Design review of the part shown in the three views and the two pictorial views. Dimensions are in mm from the part's minimum x, y and z. A direction names the side the tool comes from. Coordinates: 2 decimals unless noted, no trailing zeros. Write each loop counter-clockwise with the first axis right and the second up, starting at its lowest first coordinate (ties: lowest second). Pieces come first, ordered by that corner, then holes. Notation, with made-up numbers: M -36.75,10.5 L 0.25,10.5 A28 cw 0.25,33.5 Z; hole C 17,29.5 d5. An arc over 180 degrees is marked long. Answer as a JSON object with one key per item and string values.
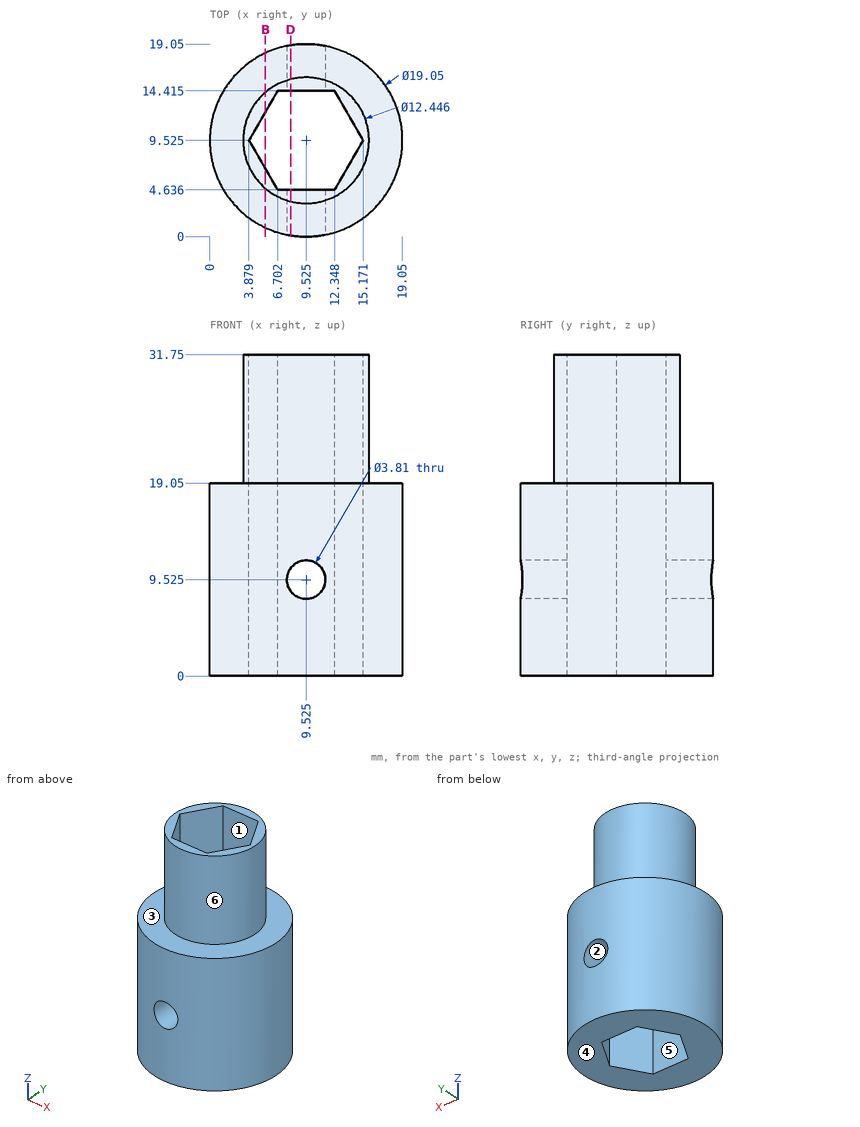
(1) Add section D-D on x = 8. Count the separate pieces of the cut face and the enclosed holes in it.
Results list:
{"separate pieces": "4", "enclosed holes": "0"}
(2) For pin 1 Ø6 at (y, z) = (2, 15) entering from -X; pin 2 Ø1 at (x, z) = (10.5, 5) entering from -Y; pin 3 Ø6 at (y, z) = (4, 18.5) entering from +X, all flat-tipped, find the tip position at first contact; note any pin that passes through.
Results list:
{"pin 1": "x = 1.14", "pin 2": "y = 0.01", "pin 3": "x = 18.71"}
(3) For the marked faces 1, 2 and 3, list the 3-axis set-ups (+Z, -Z, +X, -X, +Y, -Y) from which the entire face can be reached by the end or side of a thin tool; tool diameter is ignored.
Results list:
{"face 1": "+Z, -Z", "face 2": "+Y, -Y", "face 3": "+Z"}
(4) Wall thickness on line 1 along Z through (x, y) = (9.5, 15.5); line 2 along Z through (x, y) = (18, 6.75); line 3 along X through (y, z) = (9, 27.5) (1 decimal): over which ranges is each line inside the solid? List them lowest first. Write a range as from..to.
Results list:
{"line 1": "0..7.62, 11.43..31.75", "line 2": "0..19.05", "line 3": "3.3..4.2, 14.9..15.7"}
(5) Draft analysis for pull direction X (two halves, no side actions). For the marked faces 4, 5 and 6, state which applies: released by +X, released by -X, zero draft, split by the parting line, or undercut.
Results list:
{"face 4": "zero draft", "face 5": "undercut", "face 6": "split by the parting line"}
(6) Add section B-B on x = 5.5. Give the boundary of the cut face in (y, z).
Results list:
{"outline": "M 0.89,0 L 6.72,0 L 6.72,31.75 L 4.78,31.75 L 4.78,19.05 L 0.89,19.05 Z; M 12.33,0 L 18.16,0 L 18.16,19.05 L 14.27,19.05 L 14.27,31.75 L 12.33,31.75 Z"}
